from build123d import *

# Parameters (mm, degrees)
SURFACE_EXTRUDE1_1_DEPTH = 30
THICKEN2_T2              = 4
SURFACE_EXTRUDE2_2_DEPTH = 20
THICKEN3_T2              = 4
FILLET1_R                = 3
SKETCH3_R                = 5
CUT_EXTRUDE1_DEPTH       = 217.018517725
CUT_EXTRUDE1_DEPTH_BACK  = 217.018517725
SKETCH4_R                = 4
CUT_EXTRUDE3_DEPTH       = 10
SKETCH5_R                = 1.75
CUT_EXTRUDE4_DEPTH       = 10
CIRPATTERN1_COUNT        = 4
SKETCH6_W                = 50
SKETCH6_H                = 20
CUT_EXTRUDE5_DEPTH       = 10


with BuildPart() as body_1:
    # Surface-Extrude1: a surface, the sketch's curves swept straight by 30 mm
    with BuildLine(Plane(origin=(0, 0, 0), x_dir=(1, 0, 0), z_dir=(0, 1, 0)), mode=Mode.PRIVATE) as surface_extrude1_1_path:
        Line((-100, 30), (-100, 0))
        Line((-100, 0), (100, 0))
        Line((100, 0), (100, 30))
    surface_extrude1_1 = Shell.extrude(surface_extrude1_1_path.wire(), (0 * SURFACE_EXTRUDE1_1_DEPTH, 1 * SURFACE_EXTRUDE1_1_DEPTH, 0 * SURFACE_EXTRUDE1_1_DEPTH))
    add(Solid.thicken(surface_extrude1_1, -THICKEN2_T2))

    # Surface-Extrude2: a surface, the sketch's curves swept straight by 20 mm
    with BuildLine(Plane(origin=(0, 30, 0), x_dir=(1, 0, 0), z_dir=(0, 1, 0)), mode=Mode.PRIVATE) as surface_extrude2_2_path:
        Line((-25, 0), (25, 0))
    surface_extrude2_2 = Shell.extrude(surface_extrude2_2_path.wire(), (0 * SURFACE_EXTRUDE2_2_DEPTH, 1 * SURFACE_EXTRUDE2_2_DEPTH, 0 * SURFACE_EXTRUDE2_2_DEPTH))
    add(Solid.thicken(surface_extrude2_2, -THICKEN3_T2))

    # Fillet1
    fillet1_edges = [body_1.edges().sort_by_distance(p)[0] for p in [
        (-100, 15, 0),
        (100, 15, 0),
        (104, 15, 4),
        (-104, 15, 4),
    ]]
    fillet(fillet1_edges, radius=FILLET1_R)

    # Sketch3 → Cut-Extrude1 (cut, two sides)
    with BuildSketch(Plane(origin=(104, 0, 0), x_dir=(0, 0, -1), z_dir=(1, 0, 0))) as cut_extrude1_sk:
        with Locations((14.996831486, 15)):
            Circle(SKETCH3_R)
    extrude(amount=CUT_EXTRUDE1_DEPTH, mode=Mode.SUBTRACT)
    extrude(cut_extrude1_sk.sketch, amount=-CUT_EXTRUDE1_DEPTH_BACK, mode=Mode.SUBTRACT)

    # Sketch4 → Cut-Extrude3 (cut)
    with BuildSketch(Plane(origin=(0, 0, 0), x_dir=(-1, 0, 0), z_dir=(0, 0, -1))):
        with Locations((0, 17.2)):
            Circle(SKETCH4_R)
    extrude(amount=-CUT_EXTRUDE3_DEPTH, mode=Mode.SUBTRACT)

    # Sketch5 → Cut-Extrude4 (cut)
    with BuildSketch(Plane(origin=(0, 0, 0), x_dir=(-1, 0, 0), z_dir=(0, 0, -1))):
        with Locations((0, 25.45)):
            Circle(SKETCH5_R)
    cut_extrude4 = extrude(amount=-CUT_EXTRUDE4_DEPTH, mode=Mode.SUBTRACT)

    # CirPattern1: Cut-Extrude4 ×4 about axis
    cirpattern1_axis = Axis((0, 17.2, 0), (0, 0, 1))
    for i in range(1, CIRPATTERN1_COUNT):
        add(cut_extrude4.rotate(cirpattern1_axis, i * 360 / CIRPATTERN1_COUNT), mode=Mode.SUBTRACT)

    # Sketch6 → Cut-Extrude5 (cut)
    with BuildSketch(Plane(origin=(0, 0, 0), x_dir=(-1, 0, 0), z_dir=(0, 0, -1))):
        with Locations((0, 40)):
            Rectangle(SKETCH6_W, SKETCH6_H)
    extrude(amount=-CUT_EXTRUDE5_DEPTH, mode=Mode.SUBTRACT)


solid = body_1.part
Source: CAD feature listing. Evaluate the final solid. Frame: model axes, mm. A direction names the side the tool comes from. Give positions to 0.01 mm unless a question says otherwise; leave off trailing zeros. Order: outer loops, then holes, each group sorted by start corner. A loop starts at its lowest first (then second) coordinate and runs counter-clockwise, first axis right, second up. Notation, with made-up numbers: (33.25, -15) -> (51.25, -15) arc R17 cw to (51.25, -10) -> close; hole circle Ø8 at (-34, 57). An arc over 180 degrees is marked (long way). Write item = value, one per line.
Item 1: Contact query for flat-ended pins moving along their axis: pin 1 (3 mm diameter, centred on x = -82.5, z = -1, fed in from +Y); pin 2 (2 mm diameter, centred on x = 18.5, y = 8.5, fed in from -Z). Output: stop coordinate, or through.
Check result:
pin_1 = 30
pin_2 = 0
Item 2: Section query C-C (z = -25). Output: boundary loops of the cut face in (x, y).
Check result:
outline = (-104, 0) -> (-100, 0) -> (-100, 30) -> (-104, 30) -> close; (100, 0) -> (104, 0) -> (104, 30) -> (100, 30) -> close
Item 3: Section query A-A (y = 25.45). Output: boundary loops of the cut face in (x, z), then the cut area to 3 significant figures.
Check result:
outline = (-104, -30) -> (-100, -30) -> (-100, -3) arc R3 cw to (-97, 0) -> (-1.75, 0) -> (-1.75, 4) -> (-101, 4) arc R3 ccw to (-104, 1) -> close; (1.75, 0) -> (97, 0) arc R3 cw to (100, -3) -> (100, -30) -> (104, -30) -> (104, 1) arc R3 ccw to (101, 4) -> (1.75, 4) -> close
area = 1,060 mm²
Item 4: Section query D-D (z = -17.5). Output: boundary loops of the cut face in (x, y).
Check result:
outline = (-104, 0) -> (-100, 0) -> (-100, 10.67) -> (-104, 10.67) -> close; (-104, 19.33) -> (-100, 19.33) -> (-100, 30) -> (-104, 30) -> close; (100, 0) -> (104, 0) -> (104, 10.67) -> (100, 10.67) -> close; (100, 19.33) -> (104, 19.33) -> (104, 30) -> (100, 30) -> close
Item 5: Ray query, probe 1 along X at (y, z) = (28, -15); probe 2 along Y at (x, z) = (0, 2.35); probe 3 along Y at (x, z) = (8, 1). Return the intervals inside material, ascending.
Check result:
probe_1 = -104 to -100, 100 to 104
probe_2 = 0 to 7.2, 10.7 to 13.2, 21.2 to 23.7, 27.2 to 30
probe_3 = 0 to 15.47, 18.93 to 30
Item 6: Mould query, pull axis Z, two halves, no side actions, for faces 3 (the face through (102.03, 10.56, -17.3)), 4 (the face through (-1, 11, 0)), 5 (the face through (24, 0, 1)), 6 (the face through (-101.97, 10.56, -17.3)). Classes: +Z half, -Z half, draft (parallel to the pull), parting line (faces both ways), or undercut.
Check result:
face_3 = undercut
face_4 = -Z half
face_5 = draft
face_6 = undercut
Item 7: Section query B-B (x = 8.25). Output: boundary loops of the cut face in (y, z).
Check result:
outline = (0, 0) -> (15.45, 0) -> (15.45, 4) -> (0, 4) -> close; (18.95, 0) -> (30, 0) -> (30, 4) -> (18.95, 4) -> close
Item 8: Set-up query: faces 1 (the face through (100, 18.1, -19.3)), 2 (the face through (-9.985, 17.428, 1.972)). Return all of +Z, -Z, +X, -X, +Y, -Y with unobstructed straight access to the full face (end or side cutting, diameter ignored); none if empty.
Check result:
face_1 = -Z, +Y, -Y
face_2 = +Z, -Z
